Geometry check sheet. Reference: the model listing, model coordinates, mm. A direction names the side the tool comes from. Round coordinates to 2 decimals unless told otherwise and drop trailing zeros. Order: outer loops, then holes, each group sorted by start corner. A loop starts at its lowest first (then second) coordinate and runs counter-clockwise, first axis right, second up. Notation, with made-up numbers: M 34.5,-10 L 74.5,-10 A22 cw 74.5,9 Z; hole C 45.25,30.25 d4. An arc over 180 degrees is marked long. Answer as a JSON object with one key per item and string values. Group by question number.
```python
from build123d import *

# Parameters (mm, degrees)
SKETCH2_R           = 13
SKETCH2_R_2         = 1
BOSS_EXTRUDE2_DEPTH = 1.016
SKETCH3_R           = 13
SKETCH3_R_2         = 11.992
SKETCH3_R_3         = 10.492
SKETCH3_R_4         = 1.5
BOSS_EXTRUDE4_DEPTH = 1.016


with BuildPart() as part:
    # Sketch2 → Boss-Extrude2 (new body)
    with BuildSketch(Plane(origin=(0, 0, 0), x_dir=(1, 0, 0), z_dir=(0, 1, 0))):
        with Locations(Location((0, 0, 0), (0, 0, 270))):
            Circle(SKETCH2_R)
        with Locations(Location((0, 0, 0), (0, 0, 270))):
            Circle(SKETCH2_R_2, mode=Mode.SUBTRACT)
        with Locations(Location((4, 0, 0), (0, 0, 270))):
            Circle(SKETCH2_R_2, mode=Mode.SUBTRACT)
        with Locations(Location((8, 0, 0), (0, 0, 270))):
            Circle(SKETCH2_R_2, mode=Mode.SUBTRACT)
    extrude(amount=BOSS_EXTRUDE2_DEPTH)

    # Sketch3 → Boss-Extrude4 (add)
    # profile 1 of 2: a face of its own
    with BuildSketch(Plane(origin=(0, 1.016, 0), x_dir=(1, 0, 0), z_dir=(0, 1, 0))):
        with Locations(Location((0, 0, 0), (0, 0, 270))):
            Circle(SKETCH3_R)
        with Locations(Location((0, 0, 0), (0, 0, 270))):
            Circle(SKETCH3_R_2, mode=Mode.SUBTRACT)
    # profile 2 of 2: a face of its own
    with BuildSketch(Plane(origin=(0, 1.016, 0), x_dir=(1, 0, 0), z_dir=(0, 1, 0))):
        with Locations(Location((0, 0, 0), (0, 0, 270))):
            Circle(SKETCH3_R_3)
        with Locations(Location((0, 0, 0), (0, 0, 270))):
            Circle(SKETCH3_R_4, mode=Mode.SUBTRACT)
        with Locations(Location((4, 0, 0), (0, 0, 270))):
            Circle(SKETCH3_R_4, mode=Mode.SUBTRACT)
        with Locations(Location((8, 0, 0), (0, 0, 270))):
            Circle(SKETCH3_R_4, mode=Mode.SUBTRACT)
    extrude(amount=BOSS_EXTRUDE4_DEPTH)


solid = part.part
```
1) Sectioned sample at D-D (z = 0). Count the separate pieces of the cut face and the enclosed holes in it, then the cut area to 3 significant figures.
2) Sectioned sample at B-B (y = 0.65). Record the boundary of the cut face in (x, z).
3) Sectioned sample at C-C (z = 4.25). Record the boundary of the cut face in (x, y), then the cut area to 3 significant figures.
4) Set-up check for faces 1 (the flat face through (-9, 2.032, 9)), 2 (the cylindrical face through (6.536, 1.517, -0.325)): record each of +Z, -Z, +X, -X, +Y, -Y from which the full face is reachable in a straight line by a thin tool's end or side.
5) Release check for a two-part mould opening along X. For faces 3 (the cylindrical face through (-7.91, 1.002, -10.316)), 4 (the flat face through (-3, 0, 0)), 5 (the cylindrical face through (-0.976, 0.501, -0.217)), 6 (the cylindrical face through (4.99, 0.5, -0.13)) record: +X half, -X half, draft (parallel to the pull), parting line (faces both ways), or undercut.
6) Thickness scan on line 1 along X through (y, z) = (0.65, 0); line 2 along X through (y, z) = (1.65, 0); line 3 along X through (y, z) = (1.5, 8). Record the ranges inside material, lowest first. Write a range as [from, to].
7) Go/stop test with flat-tipped pins: P1, Ø1.8, axis at x = 4, z = 0, coming from the -Y side; P2, Ø1.5, axis at x = -0.5, z = -0.5, coming from the +Y side. Record where each tip stops, or that it passes through.
8) Sectioned sample at A-A (x = 0). Record the boundary of the cut face in (y, z).
Final values:
{
 "1": {"separate pieces": "4", "enclosed holes": "0", "area": "34.5 mm^2"},
 "2": {"outline": "C 0,0 d26; hole C 0,0 d2; hole C 4,0 d2; hole C 8,0 d2"},
 "3": {"outline": "M -12.29,0 L 12.29,0 L 12.29,2.03 L 11.21,2.03 L 11.21,1.02 L 9.59,1.02 L 9.59,2.03 L -9.59,2.03 L -9.59,1.02 L -11.21,1.02 L -11.21,2.03 L -12.29,2.03 Z", "area": "46.6 mm^2"},
 "4": {"face 1": "+Z, -Z, +X, -X, +Y", "face 2": "+Y"},
 "5": {"face 3": "parting line", "face 4": "draft", "face 5": "undercut", "face 6": "undercut"},
 "6": {"line 1": "x = [-13, -1], [1, 3], [5, 7], [9, 13]", "line 2": "x = [-13, -11.99], [-10.49, -1.5], [1.5, 2.5], [5.5, 6.5], [9.5, 10.49], [11.99, 13]", "line 3": "x = [-10.25, -8.93], [-6.79, 6.79], [8.93, 10.25]"},
 "7": {"P1": "passes through", "P2": "stops at y = 1.02"},
 "8": {"outline": "M 0,-13 L 2.03,-13 L 2.03,-11.99 L 1.02,-11.99 L 1.02,-10.49 L 2.03,-10.49 L 2.03,-1.5 L 1.02,-1.5 L 1.02,-1 L 0,-1 Z; M 0,1 L 1.02,1 L 1.02,1.5 L 2.03,1.5 L 2.03,10.49 L 1.02,10.49 L 1.02,11.99 L 2.03,11.99 L 2.03,13 L 0,13 Z"}
}
